```python
from build123d import *

# Parameters (mm, degrees)
F0_W     = 152.4
F0_H     = 76.2
F0_R     = 12.7
F1_DEPTH = 25.4
F2_T     = -2.54


with BuildPart() as f1:
    # F0 (on Front) → F1 (new body)
    with BuildSketch(Plane.XZ):
        Rectangle(F0_W, F0_H)
        with Locations((-38.1, 0)):
            Circle(F0_R, mode=Mode.SUBTRACT)
        with Locations((38.1, 0)):
            Circle(F0_R, mode=Mode.SUBTRACT)
    extrude(amount=F1_DEPTH)

    # F2
    f2_openings = [f1.faces().sort_by_distance(p)[0] for p in [
        (0, -12.7, 38.1),
        (0, -12.7, -38.1),
    ]]
    offset(amount=F2_T, openings=f2_openings)


solid = f1.part
```
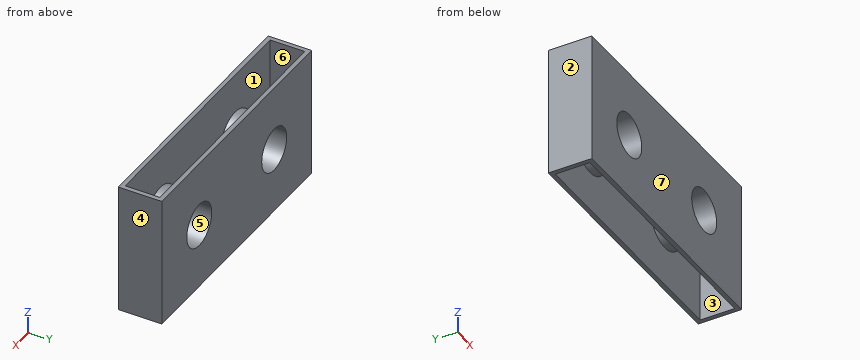
Could you check a few things on this model? Use its own coordinates, in mm. Face numbers are marked on the shaded views. A direction names the side the tool comes from. Coordinates: 2 decimals unless noted, no trailing zeros. Order: outer loops, then holes, each group sorted by start corner. A loop starts at its lowest first (then second) coordinate and runs counter-clockwise, first axis right, second up. Notation, with made-up numbers: M 22.25,-20.5 L 65.25,-20.5 A17 cw 65.25,2.5 Z; hole C 82.25,89.25 d5. An arc over 180 degrees is marked long. Use a Markdown table: item, result. Add a question column.
Q1. I want a section at B-B on x = -38.1. List the corners of the cut face in (y, z) for me, then the cut area to 3 significant figures.
Q2. I want a section at A-A on z = 0. List the corners of the cut face in (x, y) for me.
Q3. I want a section at C-C on y = -11.75. List the corners of the cut face in (x, z) for me, then the cut area to 3 significant figures.
Q4. Which directions (+Z, -Z, +X, -X, +Y, -Y) give clear straight access to the entire face, cutting with the end or side of a thin tool? Please do the marked faces 1, 2 and 3.
Q5. I want a section at D-D on z = -32.5. List the corners of the cut face in (x, y) for me.
Q6. If I drill on L1, parallel to X at y = -9, z = -22.5; L2, parallel to Y at x = 70.5, z = -23.5; L3, parallel to Z at x = 38.1, y = -19.75, over which ranges is the centre line in solid material (lowest first)?
Q7. I'm going to push a flat-ended pin straight in: pin 1 (8 mm diameter, centred on x = 47, z = -1.5, fed in from -Y). Where does the tip first touch, or does it pass through?
Q8. We'd pull the mould along X, two halves only. Please class the marked faces 4, 5, 6 and 7: pulls with the +X half, pulls with the -X half, needs draft (parallel to the pull), parting line crosses it, or undercut.
Checked values:
| question | item | result |
|---|---|---|
| 1 | outline | M -25.4,-38.1 L -22.86,-38.1 L -22.86,-15.24 L -2.54,-15.24 L -2.54,-38.1 L 0,-38.1 L 0,-12.7 L -25.4,-12.7 Z; M -25.4,12.7 L 0,12.7 L 0,38.1 L -2.54,38.1 L -2.54,15.24 L -22.86,15.24 L -22.86,38.1 L -25.4,38.1 Z |
| 1 | area | 361 mm² |
| 2 | outline | M -76.2,-25.4 L -50.8,-25.4 L -50.8,0 L -76.2,0 Z; M -25.4,-25.4 L 25.4,-25.4 L 25.4,0 L -25.4,0 Z; M 50.8,-25.4 L 76.2,-25.4 L 76.2,0 L 50.8,0 Z; hole M -73.66,-22.86 L -53.34,-22.86 L -53.34,-2.54 L -73.66,-2.54 Z; hole M -22.86,-22.86 L 22.86,-22.86 L 22.86,-2.54 L -22.86,-2.54 Z; hole M 53.34,-22.86 L 73.66,-22.86 L 73.66,-2.54 L 53.34,-2.54 Z |
| 3 | outline | M -76.2,-38.1 L -73.66,-38.1 L -73.66,38.1 L -76.2,38.1 Z; C -38.1,0 d30.48; C 38.1,0 d30.48; M 73.66,-38.1 L 76.2,-38.1 L 76.2,38.1 L 73.66,38.1 Z; hole C -38.1,0 d25.4; hole C 38.1,0 d25.4 |
| 3 | area | 833 mm² |
| 4 | face 1 | none |
| 4 | face 2 | +Z, -Z, -X, +Y, -Y |
| 4 | face 3 | +Z, -Z |
| 5 | outline | M -76.2,-25.4 L 76.2,-25.4 L 76.2,0 L -76.2,0 Z; hole M -73.66,-22.86 L 73.66,-22.86 L 73.66,-2.54 L -73.66,-2.54 Z |
| 6 | L1 | -76.2 to -73.66, 73.66 to 76.2 |
| 6 | L2 | -25.4 to -22.86, -2.54 to 0 |
| 6 | L3 | -15.24 to -12.7, 12.7 to 15.24 |
| 7 | pin 1 | y = -25.4 |
| 8 | face 4 | pulls with the +X half |
| 8 | face 5 | undercut |
| 8 | face 6 | undercut |
| 8 | face 7 | needs draft |
